Here's the drawing with two shaded views (mm, measured from the low corner). I have some questions. A direction names the side the tool comes from. Coordinates: 2 decimals unless noted, no trailing zeros. Order: outer loops, then holes, each group sorted by start corner. A loop starts at its lowest first (then second) coordinate and runs counter-clockwise, first axis right, second up. Notation, with made-up numbers: (20, -31.5) -> (51, -31.5) arc R11 ccw to (51, -14.5) -> close; hole circle Ø3 at (59.5, -30). An arc over 180 degrees is marked (long way). Answer as a JSON object with one key per item and string values. Group by question number.
(1) I want a section at A-A, the plane x = 10.7. List the corners of the cut face in (y, z) for me, plus the area to 3 significant figures.
(2) I need wall thicknesses on line 1 (Y direction, x = 36.3, z = 0.4); line 2 (Y direction, x = 21, z = 4.5); line 3 (X direction, y = 4.5, z = 9.75). Which ranges of each line are inside material? Lowest first, please.
(3) I want a section at B-B, the plane z = 7.75. List the corners of the cut face in (x, y) for me.
(4) I want a section at D-D, the plane y = 2.5. List the corners of the cut face in (x, z) for me.
(5) Which directions (+Z, -Z, +X, -X, +Y, -Y) give clear straight access to the entire face, cutting with the end or side of a thin tool? Please do the marked faces 1 and 2.
(6) I want a section at C-C, the plane y = 13. List the corners of the cut face in (x, z) for me, plus the area to 3 significant figures.
(7) For pin 1 (1.5 mm diameter, centred on x = 19.5, z = 6, fed in from -Y); pin 2 (6 mm diameter, centred on x = 11, y = 20.5, fed in from +Z); pin 3 (13 mm diameter, centred on x = 36.3, y = 13, fed in from -Z), each with a flat end and sliding along its axis, tell me the tip position at first contact or that it passes through.
(8) If we mould it in two halves opening along Y, with no side actions, what happens to the marked faces 3, 4 and 5? For each: pulls with the +Y half, pulls with the -Y half, needs draft (parallel to the pull), parting line crosses it, or undercut.
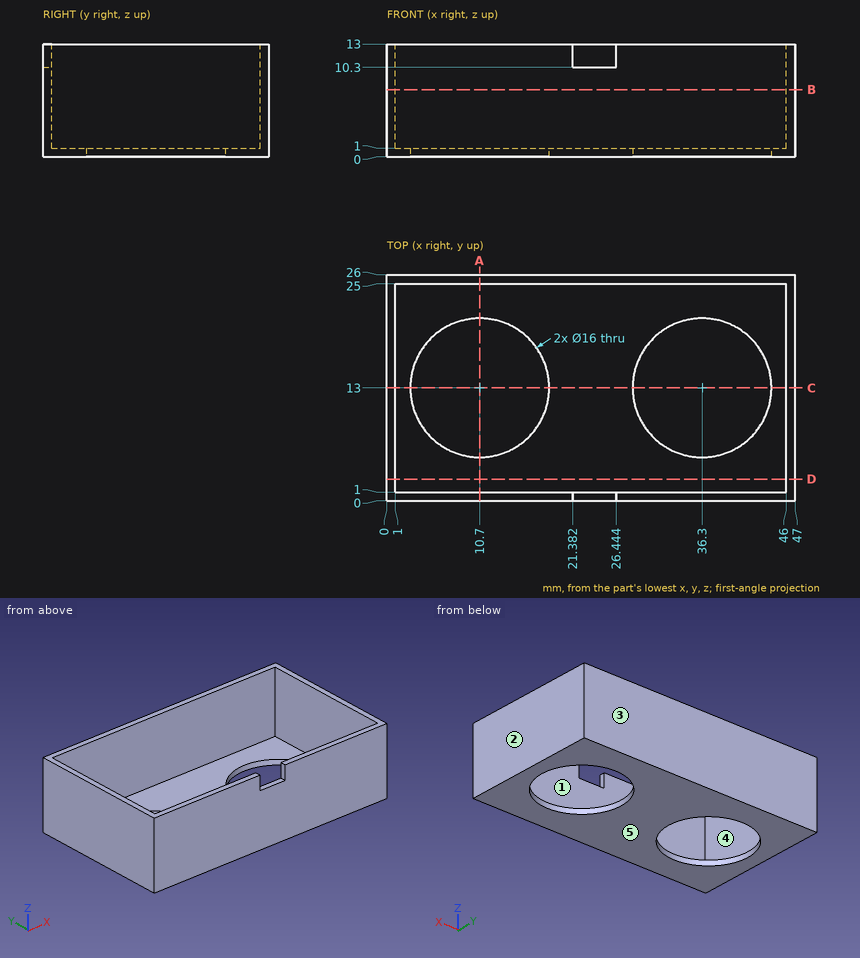
Computed values:
{
 "1": {"outline": "(0, 0) -> (5, 0) -> (5, 1) -> (1, 1) -> (1, 13) -> (0, 13) -> close; (21, 0) -> (26, 0) -> (26, 13) -> (25, 13) -> (25, 1) -> (21, 1) -> close", "area": "34.0 mm2"},
 "2": {"line 1": "y = 0 to 5, 21 to 26", "line 2": "y = 0 to 1, 25 to 26", "line 3": "x = 0 to 1, 46 to 47"},
 "3": {"outline": "(0, 0) -> (47, 0) -> (47, 26) -> (0, 26) -> close; hole (1, 1) -> (46, 1) -> (46, 25) -> (1, 25) -> close"},
 "4": {"outline": "(0, 0) -> (47, 0) -> (47, 13) -> (46, 13) -> (46, 1) -> (1, 1) -> (1, 13) -> (0, 13) -> close"},
 "5": {"face 1": "+Z", "face 2": "+Z, -Z, +X, +Y, -Y"},
 "6": {"outline": "(0, 0) -> (2.7, 0) -> (2.7, 1) -> (1, 1) -> (1, 13) -> (0, 13) -> close; (18.7, 0) -> (28.3, 0) -> (28.3, 1) -> (18.7, 1) -> close; (44.3, 0) -> (47, 0) -> (47, 13) -> (46, 13) -> (46, 1) -> (44.3, 1) -> close", "area": "39.0 mm2"},
 "7": {"pin 1": "stops at y = 0", "pin 2": "stops at z = 1", "pin 3": "passes through"},
 "8": {"face 3": "pulls with the +Y half", "face 4": "undercut", "face 5": "needs draft"}
}
